```python
from build123d import *

# Parameters (mm, degrees)
F1_DEPTH = 25.4
F3_DEPTH = 25.4
F5_R     = 6.35
F7_D     = 11.684
F7_DEPTH = 254


with BuildPart() as f1:
    # F0 (on Front) → F1 (new body)
    with BuildSketch(Plane.XZ):
        Polygon((-12.7, 0), (0, 0), (12.7, 0), (12.7, 12.7), (0, 12.7), (-12.7, 12.7), align=None)
    extrude(amount=F1_DEPTH)

    # F2 (on face) → F3 (join)
    with BuildSketch(Plane.XY.offset(12.7)):
        Polygon((7.62, -5.08), (0, -5.08), (0, -12.7), (0, -20.32), (7.62, -20.32), align=None)
        Polygon((0, -12.7), (0, -5.08), (-7.62, -5.08), (-7.62, -20.32), (0, -20.32), align=None)
    extrude(amount=F3_DEPTH)

    # F4: F1 across plane


with BuildPart() as f1_1:
    add(f1.part)
    add(f1.part.mirror(Plane.XY))

    # F5
    f5_edges = [f1_1.edges().sort_by_distance(p)[0] for p in [
        (12.7, 0, 0),
        (12.7, -25.4, 0),
        (-12.7, 0, 0),
        (-12.7, -25.4, 0),
    ]]
    fillet(f5_edges, radius=F5_R)

    # F7
    with Locations(Plane(origin=(0, 0, 0), x_dir=(-1, 0, 0), z_dir=(0, 1, 0))):
        with Locations((0, 0)):
            Hole(F7_D / 2, depth=F7_DEPTH)


solid = f1_1.part
```
Here's how the part is built. I have some questions about the finished solid (model axes, mm). A direction names the side the tool comes from. Give positions to 0.01 mm unless a question says otherwise; leave off trailing zeros. Order: outer loops, then holes, each group sorted by start corner. A loop starts at its lowest first (then second) coordinate and runs counter-clockwise, first axis right, second up. Notation, with made-up numbers: (-20, 34) -> (16, 34) arc R12 ccw to (16, 41) -> close; hole circle Ø4 at (-8.5, 25). An arc over 180 degrees is marked (long way). Use CSV: the item, a comma, the result in double quotes. Start each with the question number.
Item 1: Suppose I cut it at B-B (z = 0). List the corners of the cut face in (x, y) for me, and give its area (3 significant figures).
Item 2: Suppose I cut it at C-C (y = -9.5). List the corners of the cut face in (x, z) for me.
Item 3: Thinking about a two-plate mould opening in Z: for faces 1 (the flat face through (0, -20.32, -25)), 2 (the flat face through (0, -13, 38.1)), 3 (the cylindrical face through (-1.266, -12.878, -5.703)), 4 (the flat face through (0, -13, -38.1)), which applies, pulls with the +Z half, pulls with the -Z half, needs draft (parallel to the pull), parting line crosses it, or undercut?
Item 4: On a 3-axis mill with a long thin cutter (end or side, diameter ignored), from which of +Z, -Z, +X, -X, +Y, -Y can I reach the whole of each face in a straight line? I mean faces 5 (the flat face through (0, -5.08, -25)), 6 (the flat face through (7.62, -13, -25)), 7 (the flat face through (-7.62, -13, -25)), 8 (the flat face through (-7.62, -13, 25)), 9 (the flat face through (0, -5.08, 25)). Say none if no direction works.
Item 5: I'm going to push flat-ended pins straight in: P1, Ø12, axis at x = 2.5, z = -21, coming from the +Y side; P2, Ø7.5, axis at y = -9, z = -26, coming from the +X side; P3, Ø4.5, axis at x = -3, z = 23, coming from the -Y side. Where does each tip first touch, or does it pass through?
Item 6: Suppose I cut it at D-D (z = 11.5). List the corners of the cut face in (x, y) for me, and give its area (3 significant figures).
Item 7: If I drill on probe 1 along Z at (x, y) = (0, -14); probe 2 along Y at (x, z) = (-6.25, -25); probe 3 along X at (y, z) = (-21, -5), over which ranges is the centre line in solid material (lowest first)? Write a range as [from, to].
Item 8: Suppose I cut it at A-A (x = 0). List the corners of the cut face in (y, z) for me.
Answer block:
1,outline,"(-12.7, -19.05) arc R6.35 ccw to (-6.35, -25.4) -> (-5.84, -25.4) -> (-5.84, 0) -> (-6.35, 0) arc R6.35 ccw to (-12.7, -6.35) -> close; (5.84, -25.4) -> (6.35, -25.4) arc R6.35 ccw to (12.7, -19.05) -> (12.7, -6.35) arc R6.35 ccw to (6.35, 0) -> (5.84, 0) -> close"
1,area,"314 mm^2"
2,outline,"(-12.7, -12.7) -> (-7.62, -12.7) -> (-7.62, -38.1) -> (7.62, -38.1) -> (7.62, -12.7) -> (12.7, -12.7) -> (12.7, 12.7) -> (7.62, 12.7) -> (7.62, 38.1) -> (-7.62, 38.1) -> (-7.62, 12.7) -> (-12.7, 12.7) -> close; hole circle Ø11.68 at (0, 0)"
3,face 1,"needs draft"
3,face 2,"pulls with the +Z half"
3,face 3,"undercut"
3,face 4,"pulls with the -Z half"
4,face 5,"-Z, +X, -X, +Y"
4,face 6,"-Z, +X, +Y, -Y"
4,face 7,"-Z, -X, +Y, -Y"
4,face 8,"+Z, -X, +Y, -Y"
4,face 9,"+Z, +X, -X, +Y"
5,P1,"stops at y = -5.08"
5,P2,"stops at x = 7.62"
5,P3,"stops at y = -20.32"
6,outline,"(-12.7, -19.05) arc R6.35 ccw to (-6.35, -25.4) -> (6.35, -25.4) arc R6.35 ccw to (12.7, -19.05) -> (12.7, -6.35) arc R6.35 ccw to (6.35, 0) -> (-6.35, 0) arc R6.35 ccw to (-12.7, -6.35) -> close"
6,area,"611 mm^2"
7,probe 1,"z = [-38.1, -5.84], [5.84, 38.1]"
7,probe 2,"y = [-20.32, -5.08]"
7,probe 3,"x = [-12.39, -3.02], [3.02, 12.39]"
8,outline,"(-25.4, -12.7) -> (-20.32, -12.7) -> (-20.32, -38.1) -> (-5.08, -38.1) -> (-5.08, -12.7) -> (0, -12.7) -> (0, -5.84) -> (-25.4, -5.84) -> close; (-25.4, 5.84) -> (0, 5.84) -> (0, 12.7) -> (-5.08, 12.7) -> (-5.08, 38.1) -> (-20.32, 38.1) -> (-20.32, 12.7) -> (-25.4, 12.7) -> close"
